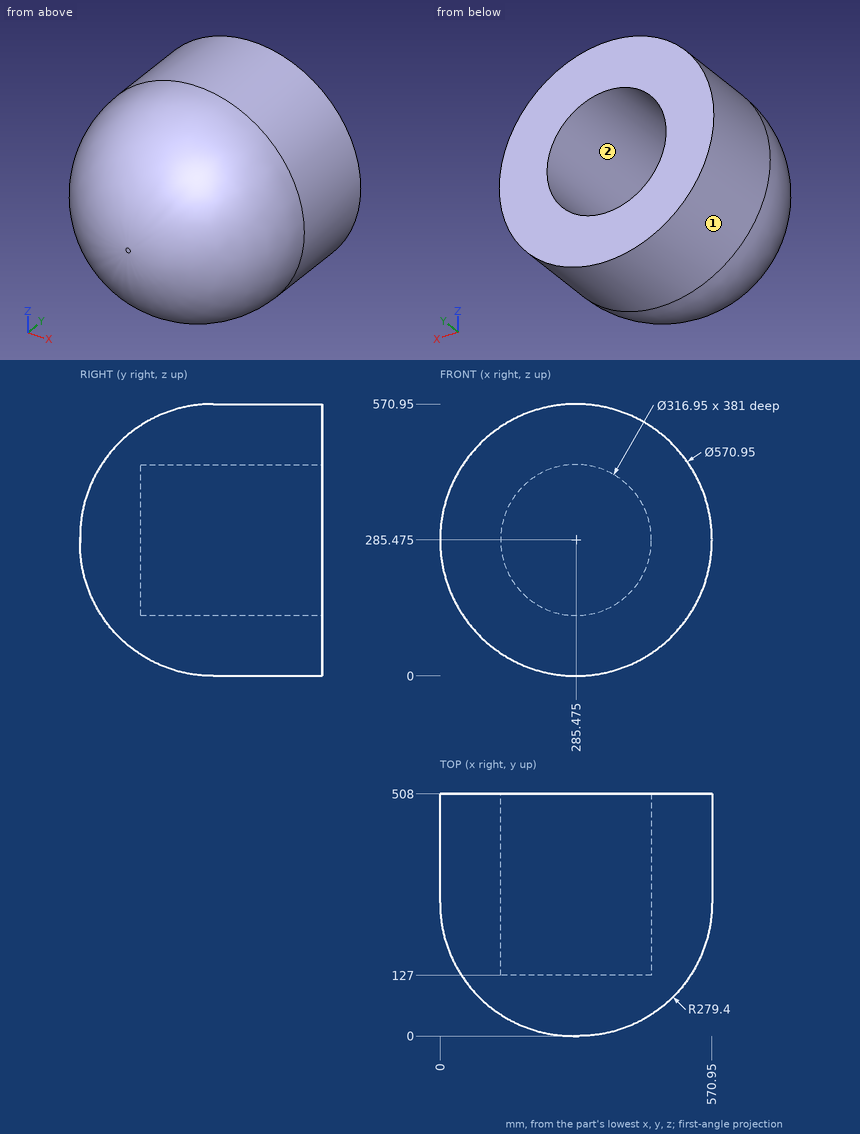
Source: three-view drawing plus pictorial views. Frame: mm from the lowest corner of the part. A direction names the side the tool comes from. Give positions to 0.01 mm unless a question says otherwise; leave off trailing zeros.
1. Pin query (flat end, axial travel): pin 1 (4 mm diameter, centred on y = 455.5, z = 338, fed in from +X); pin 2 (8 mm diameter, centred on x = 120, z = 327.5, fed in from -Y); pin 3 (3 mm diameter, centred on y = 230.5, z = 386.5, fed in from +X). Return the tip coordinate at first contact, or that it passes through.
Derived:
pin 1: stops at x = 566.44
pin 2: stops at y = 50.81
pin 3: stops at x = 548.5
2. Reachability of the marked faces 1 and 2 from +Z, -Z, +X, -X, +Y, -Y: full face, straight path, thin tool, end or side. Return the list, or none.
Derived:
face 1: +Y, -Y
face 2: +Y
3. Material intervals for L1, parallel to X at y = 190.5, z = 300.5 (1 decimal); L2, parallel to X at y = 221, z = 354; L3, parallel to Z at x = 311, y = 168.5 (1 decimal), sorted ascending.
Derived:
L1: x = 14.9 to 127.7, 443.2 to 556
L2: x = 14.71 to 142.58, 428.37 to 556.24
L3: z = 24.2 to 129.1, 441.9 to 546.8
